Drawing for the job (mm, zero at the part's lowest x, y, z). Round coordinates to 2 decimals unless told otherwise and drop trailing zeros. Loops run counter-clockwise (first coordinate to the right, second up) from the corner with the lowest first, then second, coordinate; pieces in that order, holes last. Notation, with made-up numbers: (3.25, -29) -> (58.25, -29) arc R11 cw to (58.25, -10) -> close; hole circle Ø8 at (55, 62). An arc over 180 degrees is marked (long way). Put each result on its own line as item: value. Start each with the question number.
Item 1: Pull direction Z, two halves, no side cores. Call the marked faces 1 and 2: +Z half, -Z half, draft (parallel to the pull), parting line (faces both ways), or undercut.
Item 2: Flat gauge pins, fed straight in: pin 1 Ø1.8 at (y, z) = (8, 18) entering from +X; pin 2 Ø4 at (x, z) = (19, 72.5) entering from +Y; pin 3 Ø3 at (x, y) = (21.5, 9.5) entering from -Z. Where does each tip first touch, or does it go through?
Item 3: Cut at B-B, the plane x = 15.5. List the corners of the cut face in (y, z).
Item 4: Cut at C-C, the plane z = 19.5. List the corners of the cut face in (x, y).
Item 5: Drill centre lines: probe 1 along Z at (x, y) = (4, 10); probe 2 along Y at (x, z) = (23.5, 107); probe 3 along X at (y, z) = (7, 19.5). Where is each one in solid material? Low to high. Write a range as [from, to].
Item 6: Cut at A-A, the plane y = 7.5. List the corners of the cut face in (x, z), plus the area to 3 significant figures.
Item 7: Cut at D-D, the plane z = 67. List the corners of the cut face in (x, y).
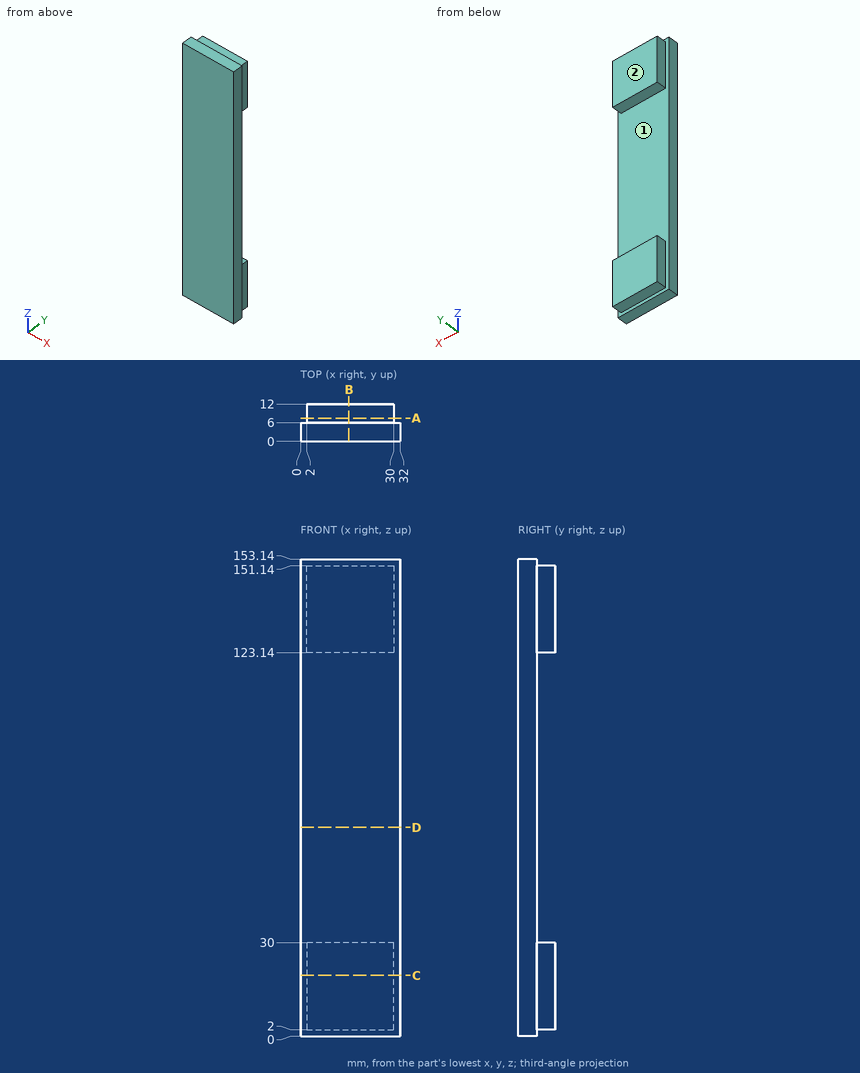
Reply:
1. face 1: undercut
1. face 2: draft
2. pin 1: stops at x = 30
2. pin 2: stops at y = 6
2. pin 3: stops at z = 2
3. outline: (0, 0) -> (6, 0) -> (6, 2) -> (12, 2) -> (12, 30) -> (6, 30) -> (6, 123.14) -> (12, 123.14) -> (12, 151.14) -> (6, 151.14) -> (6, 153.14) -> (0, 153.14) -> close
4. outline: (0, 0) -> (32, 0) -> (32, 6) -> (30, 6) -> (30, 12) -> (2, 12) -> (2, 6) -> (0, 6) -> close
5. probe 1: z = [2, 30], [123.14, 151.14]
5. probe 2: y = [0, 6]
5. probe 3: x = [2, 30]
6. outline: (2, 2) -> (30, 2) -> (30, 30) -> (2, 30) -> close; (2, 123.14) -> (30, 123.14) -> (30, 151.14) -> (2, 151.14) -> close
6. area: 1,570 mm^2
7. outline: (0, 0) -> (32, 0) -> (32, 6) -> (0, 6) -> close
